Read the model definition and answer for the solid it produces. Units are mm, in the model's axes. Face numbers are marked on the shaded views. A direction names the side the tool comes from. Give positions to 0.01 mm unless a question says otherwise; leave off trailing zeros. Loops run counter-clockwise (first coordinate to the right, second up) from the corner with the lowest first, then second, coordinate; pieces in that order, holes last. Notation, with made-up numbers: (-30.75, -36) - (12.25, -36) arc R21 ccw to (12.25, -7) - close; hole circle Ø4 at (54.5, 10.25). An arc over 180 degrees is marked (long way). Write item = value, one per line.
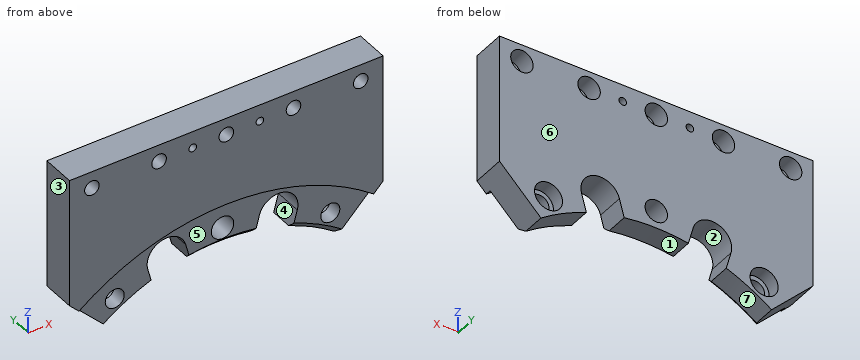
```python
from build123d import *

# Parameters (mm, degrees)
SKETCH_1_R             = 10
SKETCH_1_R_2           = 8.5
EXTRUDE_1_DEPTH        = 30
SKETCH_3_R             = 12.5
CUT_EXTRUDE_1_DEPTH    = 12
CUT_EXTRUDE_2_REACH    = 210.839
SKETCH_4_R             = 6.5
SKETCH_5_R             = 10
CUT_EXTRUDE_3_DEPTH    = 16
PATTERN_LINEAR_1_COUNT = 5
PATTERN_LINEAR_1_PITCH = 60
CUT_EXTRUDE_4_REACH    = 210.839
SKETCH_6_R             = 3.4
CUT_EXTRUDE_5_DEPTH    = 5
CHAMFER_1_SIZE         = 5


with BuildPart() as part:
    # 草图1 → 凸台-拉伸1 (new body)
    with BuildSketch(Plane(origin=(0, 0, 0), x_dir=(1, 0, 0), z_dir=(0, 1, 0))):
        with BuildLine():
            Line((-140, 0), (140, 0))
            Line((140, 0), (140, 115))
            Line((140, 115), (102.967607088, 152.032392912))
            ThreePointArc((102.967607088, 152.032392912), (83.433104198, 139.897735045), (62.490215343, 130.398149206))
            Line((62.490215343, 130.398149206), (66.726368142, 114.588611729))
            ThreePointArc((66.726368142, 114.588611729), (54.351999472, 93.155576479), (32.918964222, 105.52994515))
            Line((32.918964222, 105.52994515), (28.682811422, 121.339482627))
            ThreePointArc((28.682811422, 121.339482627), (0, 119), (-28.682811422, 121.339482627))
            Line((-28.682811422, 121.339482627), (-32.918964222, 105.52994515))
            ThreePointArc((-32.918964222, 105.52994515), (-54.351999472, 93.155576479), (-66.726368142, 114.588611729))
            Line((-66.726368142, 114.588611729), (-62.490215343, 130.398149206))
            ThreePointArc((-62.490215343, 130.398149206), (-83.433104198, 139.897735045), (-102.967607088, 152.032392912))
            Line((-102.967607088, 152.032392912), (-140, 115))
            Line((-140, 115), (-140, 0))
        make_face()
        with Locations(Location((0, 103.5, 0), (0, 0, 270))):
            Circle(SKETCH_1_R, mode=Mode.SUBTRACT)
        with Locations(Location((-96.25, 129.290109771, 0), (0, 0, 270))):
            Circle(SKETCH_1_R_2, mode=Mode.SUBTRACT)
        with Locations(Location((96.25, 129.290109771, 0), (0, 0, 90))):
            Circle(SKETCH_1_R_2, mode=Mode.SUBTRACT)
    extrude(amount=EXTRUDE_1_DEPTH)

    # 草图3 → 切除-拉伸1 (cut)
    with BuildSketch(Plane(origin=(0, 30, 0), x_dir=(1, 0, 0), z_dir=(0, 1, 0))):
        with Locations(Location((-96.25, 129.290109771, 0), (0, 0, 270))):
            Circle(SKETCH_3_R)
        with Locations(Location((96.25, 129.290109771, 0), (0, 0, 270))):
            Circle(SKETCH_3_R)
    extrude(amount=-CUT_EXTRUDE_1_DEPTH, mode=Mode.SUBTRACT)

    # 草图4 → 切除-拉伸2 (cut, up to next)
    with BuildSketch(Plane(origin=(0, 30, 0), x_dir=(1, 0, 0), z_dir=(0, 1, 0)), mode=Mode.PRIVATE) as cut_extrude_2_sk1:
        with Locations(Location((-120, 15, 0), (0, 0, 270))):
            Circle(SKETCH_4_R)
    cut_extrude_2_tool1 = extrude(cut_extrude_2_sk1.sketch, amount=-CUT_EXTRUDE_2_REACH, mode=Mode.PRIVATE) & part.part
    cut_extrude_2 = cut_extrude_2_tool1.solids().sort_by_distance((-120, 30, -15))[0]
    add(cut_extrude_2, mode=Mode.SUBTRACT)

    # 草图5 → 切除-拉伸3 (cut)
    with BuildSketch(Plane(origin=(0, 30, 0), x_dir=(1, 0, 0), z_dir=(0, 1, 0))):
        with Locations(Location((-120, 15, 0), (0, 0, 270))):
            Circle(SKETCH_5_R)
    cut_extrude_3 = extrude(amount=-CUT_EXTRUDE_3_DEPTH, mode=Mode.SUBTRACT)

    # 阵列(线性)1: 切除-拉伸2, 切除-拉伸3 ×5
    with Locations(*[(i * PATTERN_LINEAR_1_PITCH, 0, 0) for i in range(1, PATTERN_LINEAR_1_COUNT)]):
        add(cut_extrude_2, mode=Mode.SUBTRACT)
        add(cut_extrude_3, mode=Mode.SUBTRACT)

    # 草图6 → 切除-拉伸4 (cut, up to next)
    with BuildSketch(Plane(origin=(0, 30, 0), x_dir=(1, 0, 0), z_dir=(0, 1, 0)), mode=Mode.PRIVATE) as cut_extrude_4_sk1:
        with Locations(Location((-30, 15, 0), (0, 0, 270))):
            Circle(SKETCH_6_R)
    cut_extrude_4_tool1 = extrude(cut_extrude_4_sk1.sketch, amount=-CUT_EXTRUDE_4_REACH, mode=Mode.PRIVATE) & part.part
    # 草图6 → 切除-拉伸4 (cut, up to next)
    with BuildSketch(Plane(origin=(0, 30, 0), x_dir=(1, 0, 0), z_dir=(0, 1, 0)), mode=Mode.PRIVATE) as cut_extrude_4_sk2:
        with Locations(Location((30, 15, 0), (0, 0, 90))):
            Circle(SKETCH_6_R)
    cut_extrude_4_tool2 = extrude(cut_extrude_4_sk2.sketch, amount=-CUT_EXTRUDE_4_REACH, mode=Mode.PRIVATE) & part.part
    add(cut_extrude_4_tool1.solids().sort_by_distance((-30, 30, -15))[0], mode=Mode.SUBTRACT)
    add(cut_extrude_4_tool2.solids().sort_by_distance((30, 30, -15))[0], mode=Mode.SUBTRACT)

    # 草图7 → 切除-拉伸5 (cut)
    with BuildSketch(Plane.XZ):
        with BuildLine():
            Line((131.566597253, -123.433402747), (131.566597253, -152.032392912))
            Line((131.566597253, -152.032392912), (-131.566597253, -152.032392912))
            Line((-131.566597253, -152.032392912), (-131.566597253, -123.433402747))
            ThreePointArc((-131.566597253, -123.433402747), (0, -79), (131.566597253, -123.433402747))
        make_face()
    extrude(amount=-CUT_EXTRUDE_5_DEPTH, mode=Mode.SUBTRACT)

    # 倒角1
    chamfer_1_edges = [part.edges().sort_by_distance(p)[0] for p in [
        (83.433104198, 5, -139.897735045),
        (-83.433104198, 5, -139.897735045),
        (0, 5, -119),
    ]]
    chamfer(chamfer_1_edges, length=CHAMFER_1_SIZE)


solid = part.part
```
1) Each of these flat-tipped pins is pushed along its axis until it touches: P1, Ø12, axis at y = 14, z = -123, coming from the -X side; P2, Ø10, axis at y = 19.5, z = -135.5, coming from the -X side; P3, Ø10, axis at x = 77, z = -127.5, coming from the -Y side. Where does it stop, or does it pass through?
Output:
P1 = -138
P2 = -124.5
P3 = 5
2) Find the intervals of material crossed by probe 1 along X at (y, z) = (12.5, -21); probe 2 along X at (y, z) = (21, -137.5); probe 3 along X at (y, z) = (4.75, -11), in increasing order.
Output:
probe_1 = -140 to -122.5, -117.5 to -62.5, -57.5 to -2.5, 2.5 to 57.5, 62.5 to 117.5, 122.5 to 140
probe_2 = -117.5 to -105.68, -86.82 to -78.78, 78.78 to 86.82, 105.68 to 117.5
probe_3 = -140 to -125.12, -114.88 to -65.12, -54.88 to -5.12, 5.12 to 54.88, 65.12 to 114.88, 125.12 to 140
3) A cutting plane is placed at A-A on x = -120. Determine the outline of the cut face in (y, z), then the cut area to 3 significant figures.
Output:
outline = (0, -115.2) - (5, -115.2) - (5, -135) - (30, -135) - (30, -25) - (14, -25) - (14, -21.5) - (0, -21.5) - close; (0, -8.5) - (14, -8.5) - (14, -5) - (30, -5) - (30, 0) - (0, 0) - close
area = 3,450 mm²
4) The mould has two halves that part along Z. Classify the marked faces 1, 2 and 3: pulls with the +Z half, pulls with the -Z half, needs draft (parallel to the pull), parting line crosses it, or undercut.
Output:
face_1 = pulls with the -Z half
face_2 = undercut
face_3 = needs draft
5) A tool of negligible diameter and unlimited length cuts with its end or side. For the marked faces 4, 5, 6 and 7, from which of +Z, -Z, +X, -X, +Y, -Y can it reach the whole face along a straight path? Write none if from no direction.
Output:
face_4 = +Y, -Y
face_5 = -Z, -Y
face_6 = +Z, -Z, +X, -X, +Y
face_7 = -Z, +Y, -Y
6) A cutting plane is placed at B-B on y = 25.25. Give the number of separate pieces and of enclosed holes in the cut face, then the cut area to 3 significant figures.
Output:
separate_pieces = 1
enclosed_holes = 10
area = 31,600 mm²
